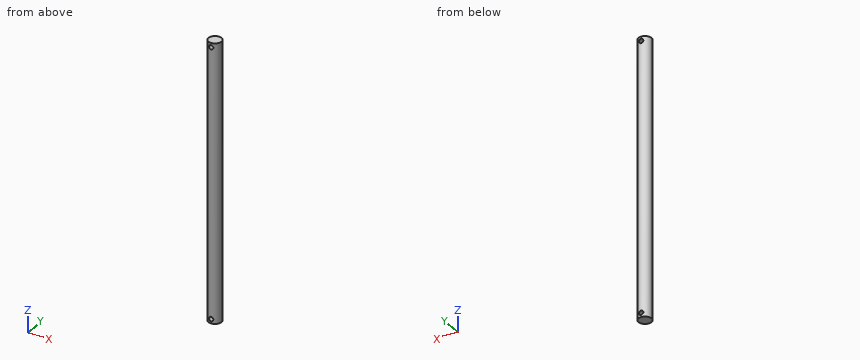
```python
from build123d import *

# Parameters (mm, degrees)
SKETCH1_R             = 4.7625
BOSS_EXTRUDE1_DEPTH   = 101.6
SKETCH2_R             = 1.5875
SPLIT_RING_HOLE_DEPTH = 102.822997464


with BuildPart() as part:
    # Sketch1 → Boss-Extrude1 (new, symmetric)
    with BuildSketch(Plane.XY):
        Circle(SKETCH1_R)
    extrude(amount=BOSS_EXTRUDE1_DEPTH, both=True)

    # Sketch2 → Split Ring Hole (cut, symmetric)
    with BuildSketch(Plane(origin=(0, 0, 0), x_dir=(1, 0, 0), z_dir=(0, 1, 0))):
        with Locations(Location((0, 98.425, 0), (0, 0, 270))):
            Circle(SKETCH2_R)
    split_ring_hole = extrude(amount=SPLIT_RING_HOLE_DEPTH, both=True, mode=Mode.SUBTRACT)

    # Mirror1: Split Ring Hole across plane
    add(split_ring_hole.mirror(Plane.XY), mode=Mode.SUBTRACT)


solid = part.part
```
Verification items for the finished model (mm, model axes). Coordinates: 2 decimals unless noted, no trailing zeros. Loops run counter-clockwise (first coordinate to the right, second up) from the corner with the lowest first, then second, coordinate; pieces in that order, holes last. Notation, with made-up numbers: (-8.75, 17) - (14.25, 17) arc R22 ccw to (14.25, 44) - close; hole circle Ø11 at (-16, 15.25). An arc over 180 degrees is marked (long way). Answer as a JSON object with one key per item and string values.
(1) Scan lines: line 1 along Z through (x, y) = (0, 3); line 2 along Z through (x, y) = (1, -1); line 3 along Y through (x, z) = (0.5, -55). Record each from-to range of solid material in increasing order.
Response:
{"line 1": "z = -101.6 to -100.01, -96.84 to 96.84, 100.01 to 101.6", "line 2": "z = -101.6 to -99.66, -97.19 to 97.19, 99.66 to 101.6", "line 3": "y = -4.74 to 4.74"}
(2) Cross-section at C-C, the plane z = 28. Record the boundary of the cut face in (x, y) (1 decimal), then the cut area to 3 significant figures.
Response:
{"outline": "circle Ø9.5 at (0, 0)", "area": "71.3 mm²"}
(3) Cross-section at A-A, the plane x = 0. Record the boundary of the cut face in (y, z), then the cut area to 4 significant figures.
Response:
{"outline": "(-4.76, -101.6) - (4.76, -101.6) - (4.76, -100.01) - (-4.76, -100.01) - close; (-4.76, -96.84) - (4.76, -96.84) - (4.76, 96.84) - (-4.76, 96.84) - close; (-4.76, 100.01) - (4.76, 100.01) - (4.76, 101.6) - (-4.76, 101.6) - close", "area": "1,875 mm²"}
(4) Cross-section at B-B, the plane y = 1.5. Record the boundary of the cut face in (x, z) (1 decimal), then the cut area to 3 significant figures.
Response:
{"outline": "(-4.5, -101.6) - (4.5, -101.6) - (4.5, 101.6) - (-4.5, 101.6) - close; hole circle Ø3.2 at (0, -98.4); hole circle Ø3.2 at (0, 98.4)", "area": "1,820 mm²"}
(5) Go/stop test with flat-tipped pins: pin 1 Ø4 at (x, z) = (-3, 37.5) entering from -Y; pin 2 Ø3 at (x, z) = (-3.5, 59) entering from +Y; pin 3 Ø2.5 at (x, z) = (0, -98.425) entering from +Y. Record where each tip stops, or that it passes through.
Response:
{"pin 1": "stops at y = -4.66", "pin 2": "stops at y = 4.32", "pin 3": "passes through"}
